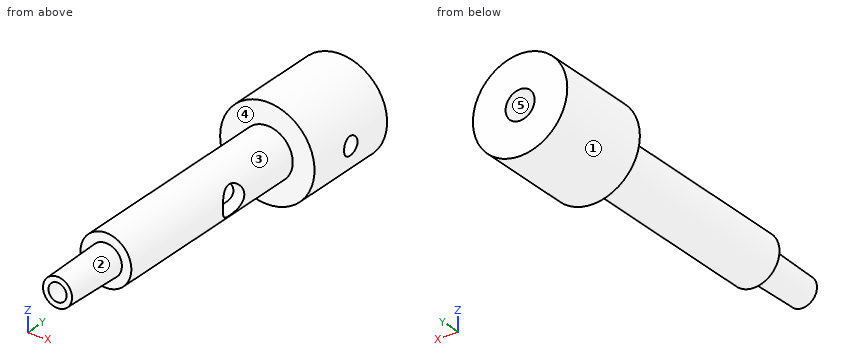
from build123d import *

# Parameters (mm, degrees)
SKETCH_2_R            = 2
CUT_EXTRUDE_1_DEPTH   = 3.5
HOLE_WIZARD_M31_D     = 2.5
HOLE_WIZARD_M31_DEPTH = 6
HOLE_WIZARD_M31_TIP   = 0.751075774


with BuildPart() as part:
    # Эскиз1 → Повернуть1 (revolve)
    with BuildSketch(Plane.XY):
        Polygon((-2, -34.780816616), (-1.25, -34.780816616), (-1.25, -19.23146208), (-2, -18.780816616), (-2, 17.719183384), (-6.5, 17.719183384), (-6.5, 4.219183384), (-3.5, 4.219183384), (-3.5, -25.780816616), (-2.2, -25.780816616), align=None)
    revolve(axis=Axis((0, 17.719183384, 0), (0, -1, 0)))

    # Эскиз2 → Вырез-Вытянуть1 (cut)
    with BuildSketch(Plane(origin=(3.5, 0, 0), x_dir=(0, 0, -1), z_dir=(1, 0, 0))):
        with Locations((0, -6.780816616)):
            Circle(SKETCH_2_R)
    extrude(amount=-CUT_EXTRUDE_1_DEPTH, mode=Mode.SUBTRACT)

    # Отверстие обработанное метчиком M31
    with Locations(Plane(origin=(6.5, 0, 0), x_dir=(0, 0, -1), z_dir=(1, 0, 0))):
        with Locations((0, 10.969183384)):
            Hole(HOLE_WIZARD_M31_D / 2, depth=HOLE_WIZARD_M31_DEPTH)
            with Locations((0, 0, -(HOLE_WIZARD_M31_DEPTH + HOLE_WIZARD_M31_TIP / 2))):  # 118° drill point
                Cone(0, HOLE_WIZARD_M31_D / 2, HOLE_WIZARD_M31_TIP, mode=Mode.SUBTRACT)


solid = part.part
Model file for the job. Use its own axes, mm. Face numbers are marked on the shaded views. A direction names the side the tool comes from. Round coordinates to 2 decimals unless told otherwise and drop trailing zeros. Order: outer loops, then holes, each group sorted by start corner. A loop starts at its lowest first (then second) coordinate and runs counter-clockwise, first axis right, second up.
(1) Pull direction Z, two halves, no side cores. Call the marked faces 3, 4 and 5: released by +Z, released by -Z, zero draft, split by the parting line, or undercut.
(2) 3-axis set-ups, long thin cutter, end or side, ignore diameter. For the marked faces 1 and 2: which of +Z, -Z, +X, -X, +Y, -Y reach the whole face in a straight line?
(3) Pin check, flat tips, straight feed: pin 1 (2 mm diameter, centred on x = -4, y = -4.5, fed in from +Z); pin 2 (1.5 mm diameter, centred on x = 0, y = -29, fed in from +Z); pin 3 (3 mm diameter, centred on x = -5, z = 2.5, fed in from -Y); pin 4 (2 mm diameter, centred on x = 0, z = 0, fed in from -Y). Stop position of each tip, or through.
(4) Band-saw the part on B-B (y = -1). List the corners of the cut face in (x, z), then the cut area to 3 significant figures.
(5) Band-saw the part on A-A (z = 0). List the corners of the cut face in (x, y).
(6) Drill centre lines: line 1 (Y direction, x = 2.75, z = 0); line 2 (X direction, y = 5, z = 0). Where is each one in solid material? Low to high.
(7) Band-saw the part on D-D (y = -20.5). List the corners of the cut face in (x, z).
(8) Band-saw the part on C-C (x = -5.5). List the corners of the cut face in (y, z).
Verdict:
1. face 3: split by the parting line
1. face 4: zero draft
1. face 5: undercut
2. face 1: +Y, -Y
2. face 2: -Y
3. pin 1: stops at z = 1.8
3. pin 2: stops at z = 2.15
3. pin 3: stops at y = 4.22
3. pin 4: passes through
4. outline: circle Ø7 at (0, 0); hole circle Ø4 at (0, 0)
4. area: 25.9 mm2
5. outline: (-6.5, 4.22) - (-3.5, 4.22) - (-3.5, -25.78) - (-2.2, -25.78) - (-2, -34.78) - (-1.25, -34.78) - (-1.25, -19.23) - (-2, -18.78) - (-2, 17.72) - (-6.5, 17.72) - close; (1.25, -34.78) - (2, -34.78) - (2.2, -25.78) - (3.5, -25.78) - (3.5, -8.78) - (2, -8.78) - (2, -18.78) - (1.25, -19.23) - close; (2, -4.78) - (3.5, -4.78) - (3.5, 4.22) - (6.5, 4.22) - (6.5, 9.72) - (2, 9.72) - close; (2, 12.22) - (6.5, 12.22) - (6.5, 17.72) - (2, 17.72) - close
6. line 1: y = -25.78 to -8.78, -4.78 to 9.72, 12.22 to 17.72
6. line 2: x = -6.5 to -2, 2 to 6.5
7. outline: circle Ø7 at (0, 0); hole circle Ø2.5 at (0, 0)
8. outline: (4.22, -3.46) - (17.72, -3.46) - (17.72, 3.46) - (4.22, 3.46) - close
